```python
from build123d import *

# Parameters (mm, degrees)
F0_R     = 10.116147
F1_DEPTH = 179.07
F0_R_2   = 18.194512
F2_DEPTH = 155.956
F0_R_3   = 35.425969
F3_DEPTH = 129.54
F0_R_4   = 46.094292
F4_DEPTH = 116.586
F0_R_5   = 50.325177
F5_DEPTH = 67.056
F6_R     = 3.896404
F7_DEPTH = 411.226


with BuildPart() as f1:
    # F0 (on Top) → F1 (new body)
    with BuildSketch(Plane.XY):
        with Locations((-71.728565, 33.039652)):
            Circle(F0_R)
    extrude(amount=F1_DEPTH)

    # F0 (on Top) → F2 (join)
    with BuildSketch(Plane.XY):
        with Locations((-71.728565, 33.039652)):
            Circle(F0_R_2)
        with Locations((-71.728565, 33.039652)):
            Circle(F0_R, mode=Mode.SUBTRACT)
    extrude(amount=F2_DEPTH)

    # F0 (on Top) → F3 (join)
    with BuildSketch(Plane.XY):
        with Locations((-71.728565, 33.039652)):
            Circle(F0_R_3)
        with Locations((-71.728565, 33.039652)):
            Circle(F0_R_2, mode=Mode.SUBTRACT)
    extrude(amount=F3_DEPTH)

    # F0 (on Top) → F4 (join)
    with BuildSketch(Plane.XY):
        with Locations((-71.728565, 33.039652)):
            Circle(F0_R_4)
        with Locations((-71.728565, 33.039652)):
            Circle(F0_R_3, mode=Mode.SUBTRACT)
    extrude(amount=F4_DEPTH)

    # F0 (on Top) → F5 (join)
    with BuildSketch(Plane.XY):
        with Locations((-71.728565, 33.039652)):
            Circle(F0_R_5)
        with Locations((-71.728565, 33.039652)):
            Circle(F0_R_4, mode=Mode.SUBTRACT)
    extrude(amount=F5_DEPTH)

    # F6 (on face) → F7 (cut)
    with BuildSketch(Plane.XY.offset(179.07)):
        with Locations((-71.728565, 33.039652)):
            Circle(F6_R)
    extrude(amount=-F7_DEPTH, mode=Mode.SUBTRACT)


solid = f1.part
```
Here's how the part is built. I have some questions about the finished solid (model axes, mm). A direction names the side the tool comes from. Coordinates: 2 decimals unless noted, no trailing zeros. Loops run counter-clockwise (first coordinate to the right, second up) from the corner with the lowest first, then second, coordinate; pieces in that order, holes last. Notation, with made-up numbers: (12.25, 5) -> (49.25, 5) arc R20 ccw to (49.25, 28) -> close; hole circle Ø11 at (-39, 26). An arc over 180 degrees is marked (long way). Return JSON: item names as keys, results as strings.
1) If we section it at A-A, the plane x = -72.5: Write out the boundary of the cut face in (y, z), then the cut area to 3 significant figures.
Results below:
{"outline": "(-17.28, 0) -> (29.22, 0) -> (29.22, 179.07) -> (22.95, 179.07) -> (22.95, 155.96) -> (14.86, 155.96) -> (14.86, 129.54) -> (-2.38, 129.54) -> (-2.38, 116.59) -> (-13.05, 116.59) -> (-13.05, 67.06) -> (-17.28, 67.06) -> close; (36.86, 0) -> (83.36, 0) -> (83.36, 67.06) -> (79.13, 67.06) -> (79.13, 116.59) -> (68.46, 116.59) -> (68.46, 129.54) -> (51.22, 129.54) -> (51.22, 155.96) -> (43.13, 155.96) -> (43.13, 179.07) -> (36.86, 179.07) -> close", "area": "12,300 mm²"}
2) If we section it at C-C, the plane x = -58.5: Write out the boundary of the cut face in (y, z).
Results below:
{"outline": "(-15.52, 0) -> (81.6, 0) -> (81.6, 67.06) -> (77.19, 67.06) -> (77.19, 116.59) -> (65.9, 116.59) -> (65.9, 129.54) -> (45.53, 129.54) -> (45.53, 155.96) -> (20.55, 155.96) -> (20.55, 129.54) -> (0.18, 129.54) -> (0.18, 116.59) -> (-11.12, 116.59) -> (-11.12, 67.06) -> (-15.52, 67.06) -> close"}
3) If we section it at D-D, the plane z = 34: Write out the boundary of the cut face in (x, y), then the cut area to 3 significant figures.
Results below:
{"outline": "circle Ø100.65 at (-71.73, 33.04); hole circle Ø7.79 at (-71.73, 33.04)", "area": "7,910 mm²"}
4) Will these pins go through, and if not, where does the flat tip stop? pin 1 (2 mm diameter, centred on x = -104, z = 85, fed in from -Y); pin 2 (7 mm diameter, centred on x = -71.73, y = 33.04, fed in from +Z); pin 3 (5 mm diameter, centred on x = -83.5, z = 91, fed in from +Y); pin 4 (5 mm diameter, centred on x = -38.5, z = 103, fed in from -Y).
Results below:
{"pin 1": "y = -0.82", "pin 2": "through", "pin 3": "y = 78.19", "pin 4": "y = -1.32"}
5) For faces 1 (the face through (-72, 29, 179.07)), 2 (the face through (-64, 25, 155.956)), which set-ups out of +Z, -Z, +X, -X, +Y, -Y let a thin tool reach every point of the face, with its end or its side?
Results below:
{"face 1": "+Z, +X, -X, +Y, -Y", "face 2": "+Z"}
6) I need wall thicknesses on line 1 (Y direction, x = -71.5, z = 119); line 2 (Z direction, x = -103, y = 71.5); line 3 (Z direction, x = -89.5, y = 57). Which ranges of each line are inside material? Lowest first, please. Write a range as from..to.
Results below:
{"line 1": "-2.39..29.15, 36.93..68.46", "line 2": "0..67.06", "line 3": "0..129.54"}
7) If we section it at B-B, the plane y = 26.5: Write out the boundary of the cut face in (x, z), then the cut area to 3 significant figures.
Results below:
{"outline": "(-121.63, 0) -> (-21.83, 0) -> (-21.83, 67.06) -> (-26.1, 67.06) -> (-26.1, 116.59) -> (-36.91, 116.59) -> (-36.91, 129.54) -> (-54.75, 129.54) -> (-54.75, 155.96) -> (-64.01, 155.96) -> (-64.01, 179.07) -> (-79.45, 179.07) -> (-79.45, 155.96) -> (-88.71, 155.96) -> (-88.71, 129.54) -> (-106.55, 129.54) -> (-106.55, 116.59) -> (-117.36, 116.59) -> (-117.36, 67.06) -> (-121.63, 67.06) -> close", "area": "13,400 mm²"}
8) Thinking about a two-plate mould opening in X: for faces 3 (the face through (-75.62, 33.21, 90.79)), 4 (the face through (-79.408, -1.544, 122.972)), 5 (the face through (-61, 34, 0)), which applies, +X half, -X half, draft (parallel to the pull), parting line (faces both ways), or undercut?
Results below:
{"face 3": "undercut", "face 4": "parting line", "face 5": "draft"}
